Autodesk Inventor part; units mm, degrees
ref_plane "YZ Plane" through (0, 0, 0) normal (1, 0, 0) x (0, 1, 0)
ref_plane "XZ Plane" through (0, 0, 0) normal (0, 1, 0) x (-1, 0, 0)
ref_plane "XY Plane" through (0, 0, 0) normal (0, 0, 1) x (1, 0, 0)
sketch "Sketch1" plane through (0, 0, 0) normal (0, 1, 0) x (-1, 0, 0)
  circle A0 centre (0, 0) radius 3.75
  circle A1 centre (0, 0) radius 6.5
  circle A2 centre (0, 0) radius 9
  dimension "d0" = 7.5
  dimension "d1" = 13
  dimension "d2" = 2.5
extrude "Extrusion1" add sketch "Sketch1" along normal blind 4 contours A1 | A2
extrude "Extrusion2" add sketch "Sketch1" against normal blind 5 contours A2
sketch "Sketch2" plane through (0, 0, 0) normal (0, -1, 0) x (1, 0, 0)
  circle A0 centre (0, 0) radius 6.5
  circle A1 centre (0, 0) radius 3.75
  circle A2 centre (0, 0) radius 9
  circle A3 centre (0, 0) radius 6.5
  line L0 (0, 6.5) -> (-1.5, 6.5)
  line L1 (-1.5, 6.5) -> (-1.5, 5.2)
  line L2 (-1.5, 5.2) -> (0, 5.2)
  line L3 (0, 5.2) -> (0, 6.5)
  line L4 (0, 6.5) -> (1.5, 6.5)
  line L5 (1.5, 6.5) -> (1.5, 5.2)
  line L6 (1.5, 5.2) -> (0, 5.2)
  arc A4 (1.5, 6.3246) -> (-1.5, 6.3246) centre (0, 0) ccw
  line L7 (-6.3792, 1.951) -> (-5.2533, 1.301)
  line L8 (-5.2533, 1.301) -> (-4.5033, 2.6)
  line L9 (-3.7533, 3.899) -> (-4.5033, 2.6)
  line L10 (-4.8792, 4.549) -> (-3.7533, 3.899)
  arc A5 (-4.7272, 4.4613) -> (-6.2272, 1.8632) centre (0, 0) ccw
  line L11 (-4.8792, -4.549) -> (-3.7533, -3.899)
  line L12 (-3.7533, -3.899) -> (-4.5033, -2.6)
  line L13 (-5.2533, -1.301) -> (-4.5033, -2.6)
  line L14 (-6.3792, -1.951) -> (-5.2533, -1.301)
  arc A6 (-6.2272, -1.8632) -> (-4.7272, -4.4613) centre (0, 0) ccw
  line L15 (1.5, -6.5) -> (1.5, -5.2)
  line L16 (1.5, -5.2) -> (0, -5.2)
  line L17 (-1.5, -5.2) -> (0, -5.2)
  line L18 (-1.5, -6.5) -> (-1.5, -5.2)
  arc A7 (-1.5, -6.3246) -> (1.5, -6.3246) centre (0, 0) ccw
  line L19 (6.3792, -1.951) -> (5.2533, -1.301)
  line L20 (5.2533, -1.301) -> (4.5033, -2.6)
  line L21 (3.7533, -3.899) -> (4.5033, -2.6)
  line L22 (4.8792, -4.549) -> (3.7533, -3.899)
  arc A8 (4.7272, -4.4613) -> (6.2272, -1.8632) centre (0, 0) ccw
  line L23 (4.8792, 4.549) -> (3.7533, 3.899)
  line L24 (3.7533, 3.899) -> (4.5033, 2.6)
  line L25 (5.2533, 1.301) -> (4.5033, 2.6)
  line L26 (6.3792, 1.951) -> (5.2533, 1.301)
  arc A9 (6.2272, 1.8632) -> (4.7272, 4.4613) centre (0, 0) ccw
  point P0 (-5.6292, 3.25)
  point P1 (-5.6292, -3.25)
  point P2 (0, -6.5)
  point P3 (5.6292, -3.25)
  point P4 (5.6292, 3.25)
  point P5 (-1.5, -6.3246)
  point P6 (1.5, -6.3246)
  point P7 (4.7272, -4.4613)
  point P8 (6.2272, -1.8632)
  point P9 (6.2272, 1.8632)
  point P10 (1.5, 6.3246)
  point P11 (-1.5, 6.3246)
  point P12 (-4.7272, 4.4613)
  point P13 (-6.2272, 1.8632)
  point P14 (-6.2272, -1.8632)
  dimension "d7" = 1.5
  dimension "d8" = 1.3
  dimension "d9" = 5.2
  dimension "d12" = 360
extrude "Extrusion3" cut sketch "Sketch2" against normal blind 4 contours L26 L25 L24 L23 A0 | A0 L22 L21 L20 L19 | L5 L6 L3 A0 | A0 L18 L17 L16 L15 | L3 L2 L1 A0 | A0 L14 L13 L12 L11 | L10 L9 L8 L7 A0
sketch "Sketch3" plane through (0, -5, 0) normal (0, -1, 0) x (1, 0, 0)
  circle A0 centre (0, 0) radius 15
  circle A1 centre (0, 0) radius 9
  circle A2 centre (0, 0) radius 6.5
  circle A3 centre (12, 0) radius 1.4
  circle A4 centre (-12, 0) radius 1.4
  dimension "d16" = 30
  dimension "d19" = 2.8
  dimension "d20" = 12
  dimension "d23" = 360
extrude "Extrusion4" add sketch "Sketch3" against normal blind 2.5 contours A0
properties part number "Potentiometer_Holder_Main"
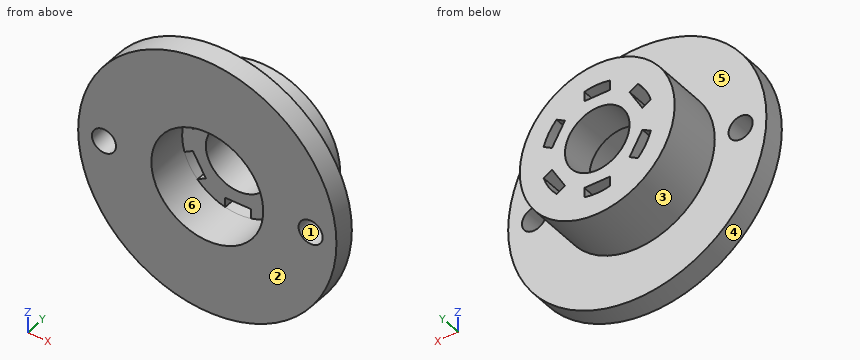
Design review of the part built by this model. Coordinates are the model's own, in mm. Face numbers are marked on the shaded views. A direction names the side the tool comes from. Coordinates: 2 decimals unless noted, no trailing zeros. Order: outer loops, then holes, each group sorted by start corner. A loop starts at its lowest first (then second) coordinate and runs counter-clockwise, first axis right, second up. Notation, with made-up numbers: M 28,89.25 L 34,89.25 A17 ccw 34,102.25 Z; hole C 27,-27.5 d10. An arc over 180 degrees is marked long. Answer as a JSON object with one key per item and string values. Group by question number.
1) Wall thickness on L1, parallel to Z at x = -6, y = 0.25; L2, parallel to Z at x = -12, y = -3.1; L3, parallel to X at y = -3.75, z = 0.5: over which ranges is each line inside the solid? List them lowest first.
2) Mouldability with a two-part tool opening along X and no side actions: class the marked faces 1, 2 and 3 as pulls with the +X half, pulls with the -X half, needs draft (parallel to the pull), parting line crosses it, or undercut.
3) Add section C-C, the plane y = -4.25. Write out the cut boundary in (x, z), then the cut area to 3 significant figures.
4) Add section D-D, the plane y = 2.5. Write out the cut boundary in (x, z), then the cut area to 3 significant figures.
5) Add section A-A, the plane x = -12. Write out the cut boundary in (y, z).
6) For pin 1 (4 mm diameter, centred on y = 0, z = -9, fed in from -X); pin 2 (10 mm diameter, centred on x = 9.5, z = -5, fed in from +Y); pin 3 (3 mm diameter, centred on x = -12, z = 0, fed in from +Y); pin 4 (0.6 mm diameter, centred on y = 1.5, z = -6, fed in from -X), all flat-tipped, find the tip position at first contact; note any pin that passes through.
7) Add section B-B, the plane z = 0. Write out the cut boundary in (x, y).
8) Tool access review of the marked faces 4, 5 and 6: name each direction out of +Z, -Z, +X, -X, +Y, -Y from which nothing blocks a thin tool from reaching the whole face with its end or side.
Computed values:
{
 "1": {"L1": "z = -6.71 to -2.5, -1.73 to 1.73, 2.5 to 6.71", "L2": "z = -9 to -1.4, 1.4 to 9", "L3": "x = -14.99 to -13.31, -10.69 to -6.48, 6.48 to 10.69, 13.31 to 14.99"},
 "2": {"face 1": "undercut", "face 2": "needs draft", "face 3": "parting line crosses it"},
 "3": {"outline": "C 0,0 d30; hole C -12,0 d2.8; hole C 0,0 d13; hole C 12,0 d2.8", "area": "562 mm^2"},
 "4": {"outline": "C 0,0 d18; hole M -6.23,-1.86 A6.5 ccw -4.73,-4.46 L -3.75,-3.9 L -5.25,-1.3 Z; hole M -6.23,1.86 L -5.25,1.3 L -3.75,3.9 L -4.73,4.46 A6.5 ccw Z; hole C 0,0 d7.5; hole M -1.5,-6.32 A6.5 ccw 1.5,-6.32 L 1.5,-5.2 L -1.5,-5.2 Z; hole M -1.5,5.2 L 1.5,5.2 L 1.5,6.32 A6.5 ccw -1.5,6.32 Z; hole M 3.75,-3.9 L 4.73,-4.46 A6.5 ccw 6.23,-1.86 L 5.25,-1.3 Z; hole M 3.75,3.9 L 5.25,1.3 L 6.23,1.86 A6.5 ccw 4.73,4.46 Z", "area": "188 mm^2"},
 "5": {"outline": "M -5,-9 L -2.5,-9 L -2.5,-1.4 L -5,-1.4 Z; M -5,1.4 L -2.5,1.4 L -2.5,9 L -5,9 Z"},
 "6": {"pin 1": "stops at x = -5.66", "pin 2": "stops at y = 4", "pin 3": "stops at y = -2.5", "pin 4": "stops at x = -6.96"},
 "7": {"outline": "M -15,-5 L -13.4,-5 L -13.4,-2.5 L -15,-2.5 Z; M -10.6,-5 L -6.5,-5 L -6.5,0 L -3.75,0 L -3.75,4 L -9,4 L -9,-2.5 L -10.6,-2.5 Z; M 3.75,0 L 6.5,0 L 6.5,-5 L 10.6,-5 L 10.6,-2.5 L 9,-2.5 L 9,4 L 3.75,4 Z; M 13.4,-5 L 15,-5 L 15,-2.5 L 13.4,-2.5 Z"},
 "8": {"face 4": "+Y, -Y", "face 5": "+Y", "face 6": "-Y"}
}
